Design review of the part built by this model. Coordinates are the model's own, in mm. Give positions to 0.01 mm unless a question says otherwise; leave off trailing zeros. Write each loop counter-clockwise with the first axis right and the second up, starting at its lowest first coordinate (ties: lowest second). Pieces come first, ordered by that corner, then holes.
```python
from build123d import *

# Parameters (mm, degrees)
F1_DEPTH = 0.508
F2_R     = 0.508
F2_R_2   = 1.143
F3_DEPTH = 0.509
F4_R     = 0.762


with BuildPart() as f1:
    # F0 (on Top) → F1 (new body)
    with BuildSketch(Plane.XY):
        with BuildLine():
            Line((-2.475686, 1.778), (-9.652, 1.778))
            ThreePointArc((-9.652, 1.778), (-10.909236, 1.257236), (-11.43, 0))
            ThreePointArc((-11.43, 0), (-10.909236, -1.257236), (-9.652, -1.778))
            Line((-9.652, -1.778), (-2.475686, -1.778))
            ThreePointArc((-2.475686, -1.778), (0, -3.048), (2.475686, -1.778))
            Line((2.475686, -1.778), (9.652, -1.778))
            ThreePointArc((9.652, -1.778), (10.909236, -1.257236), (11.43, 0))
            ThreePointArc((11.43, 0), (10.909236, 1.257236), (9.652, 1.778))
            Line((9.652, 1.778), (2.475686, 1.778))
            ThreePointArc((2.475686, 1.778), (0, 3.048), (-2.475686, 1.778))
        make_face()
    extrude(amount=F1_DEPTH)

    # F2 (on face) → F3 (cut, through all)
    with BuildSketch(Plane.XY.offset(0.508)):
        with Locations((-10.16, 0)):
            Circle(F2_R)
        with Locations((10.16, 0)):
            Circle(F2_R)
        Circle(F2_R_2)
    extrude(amount=-F3_DEPTH, mode=Mode.SUBTRACT)

    # F4
    f4_edges = [f1.edges().sort_by_distance(p)[0] for p in [
        (-2.475686, -1.778, 0.254),
        (2.475686, -1.778, 0.254),
        (-2.475686, 1.778, 0.254),
        (2.475686, 1.778, 0.254),
    ]]
    fillet(f4_edges, radius=F4_R)


solid = f1.part
```
(1) Consider section C-C, the plane x = 5.25. Give the boundary of the cut face in (y, z).
Resolved:
outline: (-1.78, 0) - (1.78, 0) - (1.78, 0.51) - (-1.78, 0.51) - close
(2) Consider section A-A, the plane z = 0.35. Give the boundary of the cut face in (x, y), then the cut area to 3 significant figures.
Resolved:
outline: (-9.65, -1.78) - (-2.84, -1.78) arc R0.76 cw to (-2.27, -2.03) arc R3.05 ccw to (2.27, -2.03) arc R0.76 cw to (2.84, -1.78) - (9.65, -1.78) arc R1.78 ccw to (9.65, 1.78) - (2.84, 1.78) arc R0.76 cw to (2.27, 2.03) arc R3.05 ccw to (-2.27, 2.03) arc R0.76 cw to (-2.84, 1.78) - (-9.65, 1.78) arc R1.78 ccw to start; hole circle Ø1.02 at (-10.16, 0); hole circle Ø2.29 at (0, 0); hole circle Ø1.02 at (10.16, 0)
area: 81.7 mm2
(3) Clearance check with flat-ended pins moving along their axes: P1, Ø0.8, axis at x = -10.16, y = 0, coming from the +Z side; P2, Ø1.3, axis at x = 10.16, y = 0, coming from the -Z side. State where each tip first meets the part, or that it passes through.
Resolved:
P1: passes through
P2: stops at z = 0
(4) Consider section B-B, the plane x = 0. Give the boundary of the cut face in (y, z), then the cut area to 3 significant figures.
Resolved:
outline: (-3.05, 0) - (-1.14, 0) - (-1.14, 0.51) - (-3.05, 0.51) - close; (1.14, 0) - (3.05, 0) - (3.05, 0.51) - (1.14, 0.51) - close
area: 1.94 mm2
(5) Consider section D-D, the plane y = 2.75. Give the boundary of the cut face in (x, z), then the cut area to 3 significant figures.
Resolved:
outline: (-1.31, 0) - (1.31, 0) - (1.31, 0.51) - (-1.31, 0.51) - close
area: 1.34 mm2
(6) To check wall thickness, follow L1, parallel to Y at x = 0, z = 0.2; L2, parallel to Y at x = 4.5, z = 0.1; L3, parallel to X at y = -0.75, z = 0.1. State the ranges of each line that lie inside material, in increasing order.
Resolved:
L1: y = -3.05 to -1.14, 1.14 to 3.05
L2: y = -1.78 to 1.78
L3: x = -11.26 to -0.86, 0.86 to 11.26
(7) Mouldability with a two-part tool opening along X and no side actions: class faces 1 (the face through (-0.036, -3.048, 0.25)), 2 (the face through (-0.2, -1.3, 0.508)), 3 (the face through (-0.248, -1.116, 0.258)) as pulls with the +X half, pulls with the -X half, needs draft (parallel to the pull), parting line crosses it, or undercut.
Resolved:
face 1: parting line crosses it
face 2: needs draft
face 3: undercut
